```python
from build123d import *

# Parameters (mm, degrees)
F0_W     = 9
F0_H     = 6
F1_DEPTH = 6
F2_W     = 6
F2_H     = 3
F3_DEPTH = 6.001
F4_R     = 0.5
F5_DEPTH = 3.001


with BuildPart() as f1:
    # F0 (on Front) → F1 (new body)
    with BuildSketch(Plane.XZ):
        Rectangle(F0_W, F0_H)
    extrude(amount=F1_DEPTH)

    # F2 (on face) → F3 (cut, through all)
    with BuildSketch(Plane.XZ.offset(6)):
        with Locations((1.5, 1.5)):
            Rectangle(F2_W, F2_H)
    extrude(amount=-F3_DEPTH, mode=Mode.SUBTRACT)

    # F4 (on face) → F5 (cut, through all)
    with BuildSketch(Plane.XY):
        with Locations((1.528993, -2.770453)):
            Circle(F4_R)
    extrude(amount=-F5_DEPTH, mode=Mode.SUBTRACT)


solid = f1.part
```
Build history of the part. All positions in model axes, mm. A direction names the side the tool comes from. Round coordinates to 2 decimals unless told otherwise and drop trailing zeros. Loops run counter-clockwise (first coordinate to the right, second up) from the corner with the lowest first, then second, coordinate; pieces in that order, holes last.
Item 1: Two-plate mould, pull along Y, no slides. Class faces 3 (the face through (1.13, -3.07, -1.48)), 4 (the face through (-4.5, -3, 0)), 5 (the face through (-1, -6, -1)): released by +Y, released by -Y, zero draft, split by the parting line, or undercut.
Item 2: Which spindle directions (+Z, -Z, +X, -X, +Y, -Y) get a long thin tool onto all of the face, cutting with end or side? Do faces 1 (the face through (1, -4, 0)), 2 (the face through (4.5, -3, -2)). Say none if no direction does.
Item 3: Pin check, flat tips, straight feed: P1, Ø1.5, axis at x = 0, y = -4.5, coming from the +Z side; P2, Ø2.5, axis at y = -3, z = 2, coming from the +X side. Stop position of each tip, or through.
Item 4: Saw through at B-B (x = -0.25). List the corners of the cut face in (y, z), then the cut area to 3 significant figures.
Item 5: Drill centre lines: line 1 along Y through (x, z) = (1.5, -0.2); line 2 along X through (y, z) = (-3.3, 0.9); line 3 along Z through (x, y) = (-1.25, -5.1). Where is each one in solid material? Low to high.
Item 6: Saw through at A-A (y = -1.55). List the corners of the cut face in (x, z), then the cut area to 3 significant figures.
Item 7: Saw through at C-C (z = 2.65). List the corners of the cut face in (x, y), then the cut area to 3 significant figures.
Worked answers:
1. face 3: undercut
1. face 4: zero draft
1. face 5: released by -Y
2. face 1: +Z, +X, +Y, -Y
2. face 2: +Z, -Z, +X, +Y, -Y
3. P1: stops at z = 0
3. P2: stops at x = -1.5
4. outline: (-6, -3) - (0, -3) - (0, 0) - (-6, 0) - close
4. area: 18.0 mm2
5. line 1: y = -6 to -3.27, -2.27 to 0
5. line 2: x = -4.5 to -1.5
5. line 3: z = -3 to 0
6. outline: (-4.5, -3) - (4.5, -3) - (4.5, 0) - (-1.5, 0) - (-1.5, 3) - (-4.5, 3) - close
6. area: 36.0 mm2
7. outline: (-4.5, -6) - (-1.5, -6) - (-1.5, 0) - (-4.5, 0) - close
7. area: 18.0 mm2
